Design review of the part built by this model. Coordinates are the model's own, in mm. A direction names the side the tool comes from. Round coordinates to 2 decimals unless told otherwise and drop trailing zeros. Loops run counter-clockwise (first coordinate to the right, second up) from the corner with the lowest first, then second, coordinate; pieces in that order, holes last. Notation, with made-up numbers: (-9.5, 65.5) - (48.5, 65.5) arc R24 cw to (48.5, 94.5) - close; hole circle Ø4 at (59.25, 17.25). An arc over 180 degrees is marked (long way). Use one line per item in the form item = value. Start each with the question number.
(1) For pin 1 (6.5 mm diameter, centred on x = 1.5, y = -0.5, fed in from -Z); pin 2 (3 mm diameter, centred on x = 3, y = -6, fed in from +Z); pin 3 (3 mm diameter, centred on x = 8, z = -4.5, fed in from +Y), all flat-tipped, find the tip position at first contact; note any pin that passes through.
(2) The part is to be moulded in two halves that separate along Y. For faces 4 (the cylindrical face through (9.481, -7.559, -5.796)), 5 (the flat face through (3.1, -1.3, 1.27)), 6 (the cylindrical face through (3.131, 0.088, -3.174)), 7 (the flat face through (12.7, 0, 0)), say which applies: released by +Y, released by -Y, zero draft, split by the parting line, or undercut.
(3) We need section D-D, the plane x = 10. Write out the cut boundary in (y, z) (3 decimals), then the cut area to 3 significant figures.
(4) We need section C-C, the plane z = 3.25. Write out the cut boundary in (x, y) (3 decimals).
(5) Machinability: for faces 1 (the cylindrical face through (2.046, -0.05, 3.776)), 2 (the cylindrical face through (3.13, 1.38, -6.2)), 3 (the flat face through (0, 0, 2)), which of the approach directions +Z, -Z, +X, -X, +Y, -Y give a long, thin tool a straight path to every point of the face, cutting with its end or side? Answer none if there is none.
(6) We need section A-A, the plane y = 0. Write out the cut boundary in (x, z) (3 decimals).
(7) Wall thickness on probe 1 along X at (y, z) = (0, 2.7); probe 2 along Z at (x, y) = (5.5, -2); probe 3 along X at (y, z) = (7.75, 2.75): over which ranges is each line inside the solid? List them lowest first. Write a range as [from, to].
(8) We need section B-B, the plane z = 0. Write out the cut boundary in (x, y) (3 decimals), then the cut area to 3 significant figures.
from build123d import *

# Parameters (mm, degrees)
F0_R     = 9.525
F1_DEPTH = 12.7
F2_R     = 9.525
F2_R_2   = 6.35
F3_DEPTH = 6.35
F5_DEPTH = 6.35
F7_D     = 2.2606
F7_DEPTH = 8.256


with BuildPart() as f1:
    # F0 (on Right) → F1 (new body)
    with BuildSketch(Plane.YZ):
        Circle(F0_R)
    extrude(amount=F1_DEPTH)

    # F2 (on face) → F3 (cut)
    with BuildSketch(Plane(origin=(0, 0, 0), x_dir=(0, -1, 0), z_dir=(-1, 0, 0))):
        Circle(F2_R)
        Circle(F2_R_2, mode=Mode.SUBTRACT)
    extrude(amount=-F3_DEPTH, mode=Mode.SUBTRACT)

    # F4 (on face) → F5 (cut)
    with BuildSketch(Plane(origin=(0, 0, 0), x_dir=(0, -1, 0), z_dir=(-1, 0, 0))):
        with BuildLine():
            Line((2.9099355663, 1.27), (-2.9099355663, 1.27))
            ThreePointArc((-2.9099355663, 1.27), (0, -3.175), (2.9099355663, 1.27))
        make_face()
    extrude(amount=-F5_DEPTH, mode=Mode.SUBTRACT)

    # F7 (through all, one way)
    with BuildSketch(Plane(origin=(0, 0, 1.27), x_dir=(1, 0, 0), z_dir=(0, 0, -1))):
        with Locations((3.175, 0)):
            Circle(F7_D / 2)
    extrude(amount=-F7_DEPTH, mode=Mode.SUBTRACT)


solid = f1.part
Data:
q1.pin_1 = -6.35
q1.pin_2 = 4.48
q1.pin_3 = 9.04
q2.face_4 = split by the parting line
q2.face_5 = undercut
q2.face_6 = undercut
q2.face_7 = zero draft
q3.outline = circle Ø19.05 at (0, 0)
q3.area = 285 mm^2
q4.outline = (0, -5.455) - (6.35, -5.455) - (6.35, -8.953) - (12.7, -8.953) - (12.7, 8.953) - (6.35, 8.953) - (6.35, 5.455) - (0, 5.455) - close; hole circle Ø2.261 at (3.175, 0)
q5.face_1 = +Z
q5.face_2 = -X
q5.face_3 = +Z, -Z, -X, +Y, -Y
q6.outline = (0, -6.35) - (6.35, -6.35) - (6.35, -9.525) - (12.7, -9.525) - (12.7, 9.525) - (6.35, 9.525) - (6.35, 6.35) - (4.305, 6.35) - (4.305, 1.27) - (6.35, 1.27) - (6.35, -3.175) - (0, -3.175) - close; (0, 1.27) - (2.045, 1.27) - (2.045, 6.35) - (0, 6.35) - close
q7.probe_1 = [0, 2.04], [4.31, 12.7]
q7.probe_2 = [-6.03, -2.47], [1.27, 6.03]
q7.probe_3 = [6.35, 12.7]
q8.outline = (0, -6.35) - (6.35, -6.35) - (6.35, -9.525) - (12.7, -9.525) - (12.7, 9.525) - (6.35, 9.525) - (6.35, 6.35) - (0, 6.35) - (0, 3.175) - (6.35, 3.175) - (6.35, -3.175) - (0, -3.175) - close
q8.area = 161 mm^2
